Autodesk Inventor part; units mm, degrees
ref_plane "YZ Plane" through (0, 0, 0) normal (1, 0, 0) x (0, 1, 0)
ref_plane "XZ Plane" through (0, 0, 0) normal (0, 1, 0) x (-1, 0, 0)
ref_plane "XY Plane" through (0, 0, 0) normal (0, 0, 1) x (1, 0, 0)
sketch "Sketch1" plane through (0, 0, 0) normal (0, 0, 1) x (1, 0, 0)
  line L0 (0, 0) -> (900, 0)
  line L1 (0, 0) -> (-900, 0)
  line L2 (0, 0) -> (0, -900)
  line L3 (0, 0) -> (0, 900)
  line L4 (-25, -25) -> (25, -25)
  line L5 (25, -25) -> (25, 25)
  line L6 (25, 25) -> (-25, 25)
  line L7 (-25, 25) -> (-25, -25)
  line L8 (-23, 23) -> (23, 23)
  line L9 (23, 23) -> (23, -23)
  line L10 (23, -23) -> (-23, -23)
  line L11 (-23, -23) -> (-23, 23)
  dimension "d0" = 900
  dimension "d1" = 900
  dimension "d2" = 900
  dimension "d3" = 900
  dimension "d4" = 25
  dimension "d5" = 25
  dimension "d6" = 25
  dimension "d7" = 25
  dimension "d9" = 2
extrude "Extrusion1" add sketch "Sketch1" against normal blind 50
extrude "Extrusion2" cut sketch "Sketch1" against normal blind 48 contours L3 L8 L9 L0 | L2 L10 L11 L1 | L0 L9 L10 L2 | L1 L11 L8 L3
fillet "Fillet1" radius 2 8 edges at (-25, -25, -25) (-25, 25, -25) (25, 25, -25) (0, 25, -50) (25, -25, -25) (25, 0, -50) (0, -25, -50) (-25, 0, -50)
properties part number "small_capsule" material "ABS Plastic"
Geometry: final body of the model. Coordinates: model frame, mm. A direction names the side the tool comes from. Coordinates: 2 decimals unless noted, no trailing zeros. Loops run counter-clockwise (first coordinate to the right, second up) from the corner with the lowest first, then second, coordinate; pieces in that order, holes last. Notation, with made-up numbers: (-1.5, 63.25) -> (7.5, 63.25) arc R14 cw to (7.5, 79.25) -> close; hole circle Ø3 at (22.5, 21.25). An arc over 180 degrees is marked (long way). Use a Markdown table: item, result. Add a question column.
(1) Section query B-B, the plane x = 20.5. Return loops of the section in (y, z), plus the area to 3 significant figures.
(2) Pin query (flat end, axial travel): pin 1 Ø12 at (x, y) = (3.5, 11) entering from +Z. Return the tip coordinate at first contact, or that it passes through.
(3) Section query A-A, the plane z = -9.5. Return loops of the section in (x, y), plus the area to 3 significant figures.
(4) Access query for faces 1 (the cylindrical face through (24.43, -24.4, -24.34)), 2 (the flat face through (0, 23, -24)). Directions: +Z, -Z, +X, -X, +Y, -Y. A direction counts if a zero-diameter tool reaches every point of the face in a straight line with its end or side. Return the directions, or none.
(5) Line query: line 1 along Y through (x, z) = (18, -27.5); line 2 along Z through (x, y) = (-17.5, -21.5). Output: solid intervals per line, ascending.
(6) Mould query, pull axis X, two halves, no side actions, for faces 3 (the flat face through (0, 0, -50)), 4 (the flat face through (0, -23, -24)), 5 (the flat face through (25, 0, -24)). Classes: pulls with the +X half, pulls with the -X half, needs draft (parallel to the pull), parting line crosses it, or undercut.
Answer:
| question | item | result |
|---|---|---|
| 1 | outline | (-25, -48) arc R2 ccw to (-23, -50) -> (23, -50) arc R2 ccw to (25, -48) -> (25, 0) -> (23, 0) -> (23, -48) -> (-23, -48) -> (-23, 0) -> (-25, 0) -> close |
| 1 | area | 290 mm^2 |
| 2 | pin 1 | stops at z = -48 |
| 3 | outline | (-25, -23) arc R2 ccw to (-23, -25) -> (23, -25) arc R2 ccw to (25, -23) -> (25, 23) arc R2 ccw to (23, 25) -> (-23, 25) arc R2 ccw to (-25, 23) -> close; hole (-23, -23) -> (23, -23) -> (23, 23) -> (-23, 23) -> close |
| 3 | area | 381 mm^2 |
| 4 | face 1 | +Z, -Z, +X, -Y |
| 4 | face 2 | +Z |
| 5 | line 1 | y = -25 to -23, 23 to 25 |
| 5 | line 2 | z = -50 to -48 |
| 6 | face 3 | needs draft |
| 6 | face 4 | undercut |
| 6 | face 5 | pulls with the +X half |
